from build123d import *

# Parameters (mm, degrees)
BOSS_EXTRUDE1_DEPTH = 1
SKETCH2_R           = 2.2
BOSS_EXTRUDE2_DEPTH = 3
CHAMFER1_SIZE       = 0.5
SKETCH4_R           = 1.95
CUT_EXTRUDE1_DEPTH  = 1
SKETCH5_R           = 0.75
CUT_EXTRUDE2_DEPTH  = 2.5
SKETCH6_R           = 6.375289794
SKETCH6_R_2         = 3.35
CUT_EXTRUDE3_DEPTH  = 133.169724505


with BuildPart() as part:
    # Sketch1 → Boss-Extrude1 (new body)
    with BuildSketch(Plane.XY):
        with BuildLine():
            Line((-129.242211844, -2.033986447), (-131.980589769, -2.033986447))
            Line((-131.980589769, -2.033986447), (-131.980589769, -4.066013553))
            Line((-131.980589769, -4.066013553), (-129.242211844, -4.066013553))
            ThreePointArc((-129.242211844, -4.066013553), (-122.699999999, -3.05), (-129.242211844, -2.033986447))
        make_face()
    extrude(amount=-BOSS_EXTRUDE1_DEPTH)

    # Sketch2 → Boss-Extrude2 (add)
    with BuildSketch(Plane(origin=(0, 0, -1), x_dir=(-1, 0, 0), z_dir=(0, 0, -1))):
        with Locations((126.049999999, -3.05)):
            Circle(SKETCH2_R)
    extrude(amount=BOSS_EXTRUDE2_DEPTH)

    # Chamfer1
    chamfer1_edges = [part.edges().sort_by_distance(p)[0] for p in [
        (-123.849999999, -3.05, -4),
    ]]
    chamfer(chamfer1_edges, length=CHAMFER1_SIZE)

    # Sketch4 → Cut-Extrude1 (cut)
    with BuildSketch(Plane.XY):
        with Locations((-126.049999999, -3.05)):
            Circle(SKETCH4_R)
    extrude(amount=-CUT_EXTRUDE1_DEPTH, mode=Mode.SUBTRACT)

    # Sketch5 → Cut-Extrude2 (cut)
    with BuildSketch(Plane.XY.offset(-1)):
        with Locations((-126.049999999, -3.05)):
            Circle(SKETCH5_R)
    extrude(amount=-CUT_EXTRUDE2_DEPTH, mode=Mode.SUBTRACT)

    # Sketch6 → Cut-Extrude3 (cut, through all)
    with BuildSketch(Plane(origin=(0, 0, -1), x_dir=(-1, 0, 0), z_dir=(0, 0, -1))):
        with Locations((126.049999999, -3.05)):
            Circle(SKETCH6_R)
        with Locations(Location((126.049999999, -3.05, 0), (0, 0, 180))):
            Circle(SKETCH6_R_2, mode=Mode.SUBTRACT)
    extrude(amount=-CUT_EXTRUDE3_DEPTH, mode=Mode.SUBTRACT)


solid = part.part
Input: part model. Units: mm. Frame: model coordinates. A direction names the side the tool comes from. Give positions to 0.01 mm unless a question says otherwise; leave off trailing zeros. Loops run counter-clockwise (first coordinate to the right, second up) from the corner with the lowest first, then second, coordinate; pieces in that order, holes last. Notation, with made-up numbers: M -12.5,16 L 42.5,16 A22 ccw 42.5,22 Z; hole C 5.25,63.5 d7. An arc over 180 degrees is marked long. Use one line per item in the form item = value.
1. Section query D-D, the plane z = -3.6. Return the cut outline in (x, y), and give its area (3 significant figures).
Numbers:
outline = C -126.05,-3.05 d4.2
area = 13.9 mm²
2. First-contact query: pin 1 (1.2 mm diameter, centred on x = -125.5, y = -3.5, fed in from +Z); pin 2 (2 mm diameter, centred on y = -1.5, z = -2.5, fed in from -X); pin 3 (2 mm diameter, centred on y = -4.5, z = -0.5, fed in from +X). Flat tips, straight axial feed; report the tip coordinate or a pass-through.
Numbers:
pin_1 = -1
pin_2 = -128.18
pin_3 = -122.73
3. Section query B-B, the plane y = -3.05. Return the cut outline in (x, z), and give its area (3 significant figures).
Numbers:
outline = M -129.4,-1 L -128.25,-1 L -128.25,-3.5 L -127.75,-4 L -124.35,-4 L -123.85,-3.5 L -123.85,-1 L -122.7,-1 L -122.7,0 L -124.1,0 L -124.1,-1 L -125.3,-1 L -125.3,-3.5 L -126.8,-3.5 L -126.8,-1 L -128,-1 L -128,0 L -129.4,0 Z
area = 12.0 mm²
4. Section query A-A, the plane x = -126.05. Return the cut outline in (y, z), and give its area (3 significant figures).
Numbers:
outline = M -6.4,-1 L -5.25,-1 L -5.25,-3.5 L -4.75,-4 L -1.35,-4 L -0.85,-3.5 L -0.85,-1 L 0.3,-1 L 0.3,0 L -1.1,0 L -1.1,-1 L -2.3,-1 L -2.3,-3.5 L -3.8,-3.5 L -3.8,-1 L -5,-1 L -5,0 L -6.4,0 Z
area = 12.0 mm²
5. Pull-direction query (X, two-part tool) for faces 1 (the face through (-126.8, -3, -2.2)), 2 (the face through (-123.852, -2.953, -2.232)), 3 (the face through (-123.9, -3, 0)); classes: released by +X, released by -X, zero draft, split by the parting line, or undercut.
Numbers:
face_1 = undercut
face_2 = split by the parting line
face_3 = zero draft
6. Line query: L1, parallel to Y at x = -126.05, z = -0.3; L2, parallel to Y at x = -126.05, z = -1.75; L3, parallel to Y at x = -128, z = -1.2. Output: solid intervals per line, ascending.
Numbers:
L1 = -6.4 to -5, -1.1 to 0.3
L2 = -5.25 to -3.8, -2.3 to -0.85
L3 = -4.07 to -2.03
7. Section query C-C, the plane z = -1.8. Return the cut outline in (x, y), and give its area (3 significant figures).
Numbers:
outline = C -126.05,-3.05 d4.4; hole C -126.05,-3.05 d1.5
area = 13.4 mm²
8. Reachability of faces 4 (the face through (-126, -4, -1)), 5 (the face through (-126, -3, -4)) from +Z, -Z, +X, -X, +Y, -Y: full face, straight path, thin tool, end or side. Return the list, or none.
Numbers:
face_4 = +Z
face_5 = -Z, +X, -X, +Y, -Y
